```python
from build123d import *

# Parameters (mm, degrees)
BOSS_EXTRUDE1_DEPTH = 12
BOSS_EXTRUDE2_DEPTH = 2
BOSS_EXTRUDE3_DEPTH = 2


with BuildPart() as part:
    # Sketch1 → Boss-Extrude1 (new body)
    with BuildSketch(Plane(origin=(0, 0, 0), x_dir=(1, 0, 0), z_dir=(0, 1, 0))):
        Polygon((109.556624327, -4.42820323), (-109.556624327, -4.42820323), (-112.113248654, 0), (-2.556624327, 189.75763964), (2.556624327, 189.75763964), (112.113248654, 0), align=None)
        Polygon((-107.824573519, -1.42820323), (-108.649147039, 0), (-99.473720558, 15.892304845), (-89.473720558, -1.42820323), align=None, mode=Mode.SUBTRACT)
        Polygon((-0.824573519, 186.75763964), (0.824573519, 186.75763964), (10, 170.865334795), (-10, 170.865334795), align=None, mode=Mode.SUBTRACT)
        Polygon((108.649147039, 0), (107.824573519, -1.42820323), (89.473720558, -1.42820323), (99.473720558, 15.892304845), align=None, mode=Mode.SUBTRACT)
        Polygon((-11.732050808, 167.865334795), (11.732050808, 167.865334795), (97.741669751, 18.892304845), (86.009618943, -1.42820323), (-86.009618943, -1.42820323), (-97.741669751, 18.892304845), align=None, mode=Mode.SUBTRACT)
    extrude(amount=BOSS_EXTRUDE1_DEPTH)

    # Sketch1_4 → Boss-Extrude2 (add)
    with BuildSketch(Plane(origin=(0, 0, 0), x_dir=(1, 0, 0), z_dir=(0, 1, 0))):
        Polygon((-97.741669751, 18.892304845), (-11.732050808, 167.865334795), (11.732050808, 167.865334795), (97.741669751, 18.892304845), (86.009618943, -1.42820323), (-86.009618943, -1.42820323), align=None)
        Polygon((-10.288675135, 165.365334795), (-94.854918405, 18.892304845), (-84.56624327, 1.07179677), (84.56624327, 1.07179677), (94.854918405, 18.892304845), (10.288675135, 165.365334795), align=None, mode=Mode.SUBTRACT)
    extrude(amount=BOSS_EXTRUDE2_DEPTH)

    # Sketch2 → Boss-Extrude3 (add)
    with BuildSketch(Plane.XZ):
        Polygon((101.205771366, -18.892304845), (87.741669751, 4.42820323), (-87.741669751, 4.42820323), (-101.205771366, -18.892304845), (-13.464101615, -170.865334795), (13.464101615, -170.865334795), align=None)
        Polygon((-11.732050807, -167.865334795), (11.732050807, -167.865334795), (97.741669751, -18.892304845), (86.009618943, 1.42820323), (-86.009618943, 1.42820323), (-97.741669751, -18.892304845), align=None, mode=Mode.SUBTRACT)
    extrude(amount=BOSS_EXTRUDE3_DEPTH)


solid = part.part
```
CAD build for the part. Positions are in the model's coordinates, mm. A direction names the side the tool comes from. Round coordinates to 2 decimals unless told otherwise and drop trailing zeros. Loops run counter-clockwise (first coordinate to the right, second up) from the corner with the lowest first, then second, coordinate; pieces in that order, holes last. Notation, with made-up numbers: M -2.75,86.25 L 52.25,86.25 A20 cw 52.25,104.25 Z; hole C -29.5,66 d2. An arc over 180 degrees is marked long. Use a Markdown table: item, result. Add a question column.
(1) Flat gauge pins, fed straight in: pin 1 (3.5 mm diameter, centred on x = -102, y = 7.5, fed in from -Z); pin 2 (5 mm diameter, centred on x = 27.5, y = 7.5, fed in from -Z); pin 3 (3 mm diameter, centred on y = 2, z = -107, fed in from +X). Where does each tip first touch, or does it go through?
(2) Cut at A-A (y = 5). Give the cut face in (x, z), and give its area (3 significant figures).
(3) Drill centre lines: line 1 (Z direction, x = 5, y = -1.25); line 2 (X direction, y = 8.25, z = -160.5); line 3 (Y direction, x = -87, z = -33). Where is each one in solid material? Low to high.
(4) Pull direction Z, two halves, no side cores. Call faces 1 (the face through (-8, -2, 2)), 2 (the face through (0, 6, -189.758)), 3 (the face through (0, 5, -170.865)): +Z half, -Z half, draft (parallel to the pull), parting line (faces both ways), or undercut.
(5) Which spindle directions (+Z, -Z, +X, -X, +Y, -Y) get a long thin tool onto all of the face, cutting with end or side? Do faces 4 (the face through (54.135, -0.986, -94.422)), 5 (the face through (1, 7, 1.428)), 6 (the face through (89.64, 0.99, -9.86)). Say none if no direction does.
(6) Cut at B-B (z = -33). Give the cut face in (x, y), and give its area (3 significant figures).
(7) Cut at C-C (x = -33.5). Give the cut face in (y, z), and give its area (3 significant figures).
Geometry says:
| question | item | result |
|---|---|---|
| 1 | pin 1 | stops at z = -20.55 |
| 1 | pin 2 | stops at z = -150.88 |
| 1 | pin 3 | stops at x = 51.2 |
| 2 | outline | M -112.11,0 L -2.56,-189.76 L 2.56,-189.76 L 112.11,0 L 109.56,4.43 L -109.56,4.43 Z; hole M -108.65,0 L -99.47,-15.89 L -89.47,1.43 L -107.82,1.43 Z; hole M -97.74,-18.89 L -11.73,-167.87 L 11.73,-167.87 L 97.74,-18.89 L 86.01,1.43 L -86.01,1.43 Z; hole M -10,-170.87 L -0.82,-186.76 L 0.82,-186.76 L 10,-170.87 Z; hole M 89.47,1.43 L 99.47,-15.89 L 108.65,0 L 107.82,1.43 Z |
| 2 | area | 2,180 mm² |
| 3 | line 1 | z = -170.87 to -167.87, 1.43 to 4.43 |
| 3 | line 2 | x = -19.45 to -15.98, 15.98 to 19.45 |
| 3 | line 3 | y = 0 to 2 |
| 4 | face 1 | draft |
| 4 | face 2 | -Z half |
| 4 | face 3 | undercut |
| 5 | face 4 | -Y |
| 5 | face 5 | +Y |
| 5 | face 6 | +Y, -Y |
| 6 | outline | M -93.06,-2 L -89.6,-2 L -89.6,0 L -86.71,0 L -86.71,2 L -89.6,2 L -89.6,12 L -93.06,12 Z; M 86.71,0 L 89.6,0 L 89.6,-2 L 93.06,-2 L 93.06,12 L 89.6,12 L 89.6,2 L 86.71,2 Z |
| 6 | area | 109 mm² |
| 7 | outline | M -2,-136.16 L 12,-136.16 L 12,-130.16 L 2,-130.16 L 2,-125.16 L 0,-125.16 L 0,-130.16 L -2,-130.16 Z; M -2,1.43 L 0,1.43 L 0,-1.07 L 2,-1.07 L 2,1.43 L 12,1.43 L 12,4.43 L -2,4.43 Z |
| 7 | area | 141 mm² |
